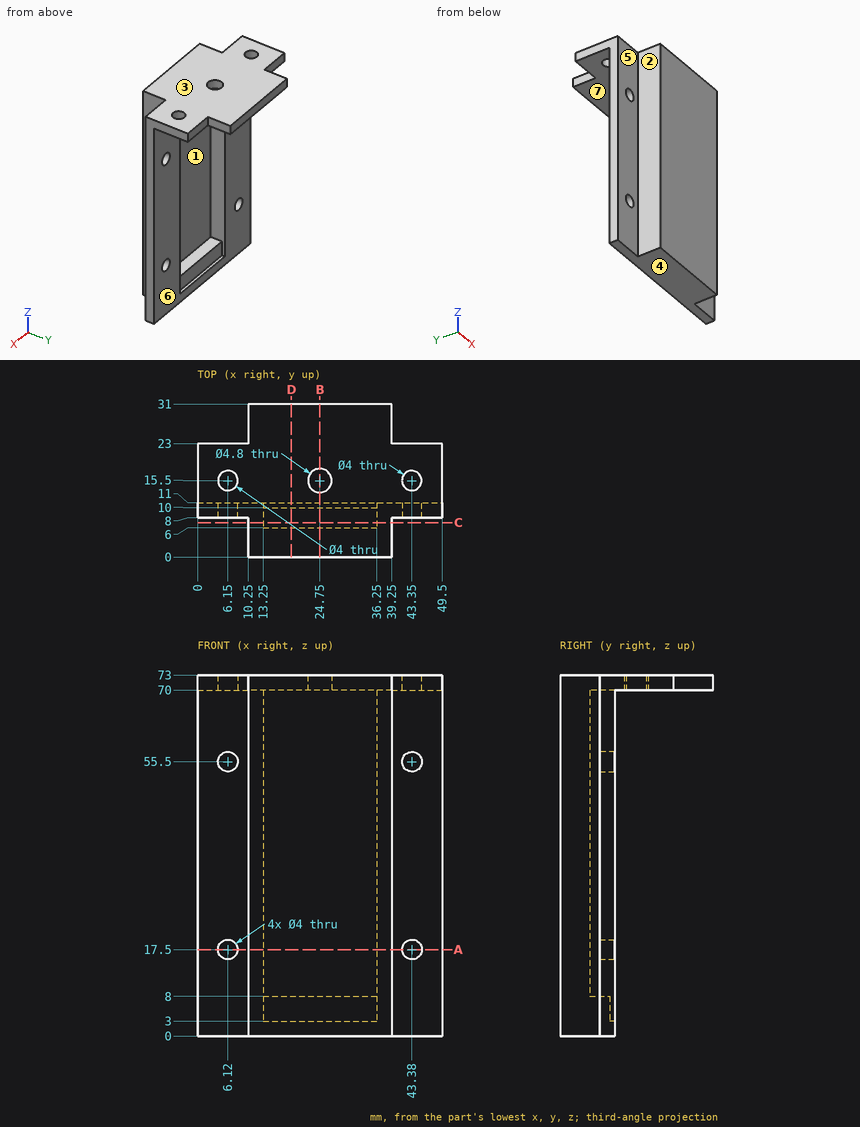
Geometry: see drawing. Coordinates: mm, zero at the bounding-box minimum. A direction names the side the tool comes from. Give positions to 0.01 mm unless a question says otherwise; leave off trailing zeros. Order: outer loops, then holes, each group sorted by start corner. A loop starts at its lowest first (then second) coordinate and runs counter-clockwise, first axis right, second up. Notation, with made-up numbers: M 89.25,21.5 L 109.25,21.5 A26 cw 109.25,38.5 Z; hole C 79,83 d4. An arc over 180 degrees is marked long. Answer as CSV lines item,"result". Start each with the question number.
1) Line query: line 1 (X direction, y = 9.5, z = 16); line 2 (Y direction, x = 43.35, z = 70.8); line 3 (Z direction, x = 3.5, y = 15.5). Output: solid intervals per line, ascending. Write a range as from..to.
2) Cut plane B-B (x = 24.75). Output: boundary loops of the cut face in (y, z).
3) Cut plane D-D (x = 19). Output: boundary loops of the cut face in (y, z).
4) Cut plane A-A (z = 17.5). Output: boundary loops of the cut face in (x, y), then the cut area to 4 significant figures.
5) Cut plane C-C (y = 7). Output: boundary loops of the cut face in (x, z).
6) Set-up query: the marked faces 5, 6 and 7. Return all of +Z, -Z, +X, -X, +Y, -Y with unobstructed straight access to the full face (end or side cutting, diameter ignored); none if empty.
7) First-contact query: P1, Ø1.5, axis at x = 19.5, y = 17, coming from the -Z side; P2, Ø6.5, axis at y = 4.5, z = 37, coming from the +X side; P3, Ø6.5, axis at x = 6.12, z = 17.5, coming from the +Y side. Flat tips, straight axial feed; report the tip coordinate or a pass-through.
8) Mould query, pull axis Z, two halves, no side actions, for the marked faces 1, 2, 3 and 4. Classes: +Z half, -Z half, draft (parallel to the pull), parting line (faces both ways), or undercut.
Findings below:
1,line 1,"x = 0..4.8, 7.44..13.25, 36.25..42.06, 44.7..49.5"
1,line 2,"y = 8..13.5, 17.5..23"
1,line 3,"z = 70..73"
2,outline,"M 0,0 L 11,0 L 11,3 L 10,3 L 10,8 L 6,8 L 6,70 L 13.1,70 L 13.1,73 L 0,73 Z; M 17.9,70 L 31,70 L 31,73 L 17.9,73 Z"
3,outline,"M 0,0 L 11,0 L 11,3 L 10,3 L 10,8 L 6,8 L 6,70 L 31,70 L 31,73 L 0,73 Z"
4,outline,"M 0,8 L 4.12,8 L 4.12,11 L 0,11 Z; M 8.12,8 L 10.25,8 L 10.25,0 L 39.25,0 L 39.25,8 L 41.38,8 L 41.38,11 L 36.25,11 L 36.25,6 L 13.25,6 L 13.25,11 L 8.12,11 Z; M 45.38,8 L 49.5,8 L 49.5,11 L 45.38,11 Z"
4,area,"241.5 mm²"
5,outline,"M 10.25,0 L 39.25,0 L 39.25,73 L 10.25,73 Z; hole M 13.25,8 L 36.25,8 L 36.25,70 L 13.25,70 Z"
6,face 5,"+Z, -Z, -X, -Y"
6,face 6,"-Z, +X, -X, +Y"
6,face 7,"+Y"
7,P1,"stops at z = 70"
7,P2,"stops at x = 39.25"
7,P3,"stops at y = 11"
8,face 1,"undercut"
8,face 2,"draft"
8,face 3,"+Z half"
8,face 4,"-Z half"
